Geometry check sheet. Reference: the model listing, model coordinates, mm. A direction names the side the tool comes from. Coordinates: 2 decimals unless noted, no trailing zeros. Write each loop counter-clockwise with the first axis right and the second up, starting at its lowest first coordinate (ties: lowest second). Pieces come first, ordered by that corner, then holes. Notation, with made-up numbers: (11, 37.25) - (18, 37.25) arc R27 cw to (18, 54.25) - close; hole circle Ø1 at (-24.5, 16). An arc over 180 degrees is marked (long way). Answer as a JSON object with one key per item and string values. Group by question number.
from build123d import *

# Parameters (mm, degrees)
SKETCH1_R           = 11.9
SKETCH1_W           = 2.4
SKETCH1_H           = 5
BOSS_EXTRUDE2_DEPTH = 2
SKETCH2_W           = 2.1
SKETCH2_H           = 2.4
BOSS_EXTRUDE3_DEPTH = 4.7
SKETCH4_W           = 2.1
SKETCH4_H           = 2.3
BOSS_EXTRUDE5_DEPTH = 1
SKETCH5_W           = 2.1
SKETCH5_H           = 2.3
BOSS_EXTRUDE6_DEPTH = 1
CHAMFER1_SIZE       = 1


with BuildPart() as part:
    # Sketch1 → Boss-Extrude2 (new body)
    with BuildSketch(Plane.XY):
        Circle(SKETCH1_R)
        with Locations((10, 0)):
            Rectangle(SKETCH1_W, SKETCH1_H, mode=Mode.SUBTRACT)
    extrude(amount=BOSS_EXTRUDE2_DEPTH)

    # Sketch2 → Boss-Extrude3 (add)
    with BuildSketch(Plane.XY.offset(2)):
        with Locations((-10, 0)):
            Rectangle(SKETCH2_W, SKETCH2_H)
    extrude(amount=BOSS_EXTRUDE3_DEPTH)

    # Sketch4 → Boss-Extrude5 (add)
    with BuildSketch(Plane(origin=(0, 1.2, 0), x_dir=(1, 0, 0), z_dir=(0, 1, 0))):
        with Locations((-10, -5.55)):
            Rectangle(SKETCH4_W, SKETCH4_H)
    extrude(amount=BOSS_EXTRUDE5_DEPTH)

    # Sketch5 → Boss-Extrude6 (add)
    with BuildSketch(Plane.XZ.offset(1.2)):
        with Locations((-10, 5.55)):
            Rectangle(SKETCH5_W, SKETCH5_H)
    extrude(amount=BOSS_EXTRUDE6_DEPTH)

    # Chamfer1
    chamfer1_edges = [part.edges().sort_by_distance(p)[0] for p in [
        (-8.95, 0, 6.7),
        (-11.05, 0, 6.7),
        (-10, 2.2, 6.7),
        (-10, -2.2, 6.7),
    ]]
    chamfer(chamfer1_edges, length=CHAMFER1_SIZE)


solid = part.part
(1) Section check C-C (x = 9.5). Record the cut outline in (y, z), and give its area (3 significant figures).
(2) Section check B-B (z = 1.25). Record the cut outline in (x, y).
(3) Section check D-D (x = 0). Record the cut outline in (y, z), and give its area (3 significant figures).
(4) Draft check along Z on faces 1 (the face through (-10, -2, 4.4)), 2 (the face through (-9.46, -0.03, 6.21)), 3 (the face through (8.8, 0, 1)). Enter one of: +Z half, -Z half, draft (parallel to the pull), parting line (faces both ways), or undercut.
(5) Material ranges on L1, parallel to Z at x = -3.5, y = 3; L2, parallel to Y at x = 0.25, z = 0.5; L3, parallel to X at y = -7.25, z = 1.75, recorded low to high. Write a range as [from, to].
(6) Set-up check for faces 4 (the face through (-10, -1.2, 3)), 5 (the face through (-11.05, 0, 4)), 6 (the face through (-8.95, 0, 4)): record each of +Z, -Z, +X, -X, +Y, -Y from which the full face is reachable in a straight line by a thin tool's end or side.
(7) Gauge pin test, flat ends, axial feed: pin 1 (1 mm diameter, centred on y = 1, z = 1, fed in from -X); pin 2 (2.5 mm diameter, centred on x = -9.5, z = 3, fed in from -Y); pin 3 (2 mm diameter, centred on x = 5, z = 2, fed in from -Y); pin 4 (2 mm diameter, centred on x = 8.5, z = 4.5, fed in from -Y). Record the tip position at first contact, or that the pin passes through.
(8) Section check A-A (y = 0). Record the cut outline in (x, z).
Conclusion:
{
 "1": {"outline": "(-7.17, 0) - (-2.5, 0) - (-2.5, 2) - (-7.17, 2) - close; (2.5, 0) - (7.17, 0) - (7.17, 2) - (2.5, 2) - close", "area": "18.7 mm^2"},
 "2": {"outline": "circle Ø23.8 at (0, 0); hole (8.8, -2.5) - (11.2, -2.5) - (11.2, 2.5) - (8.8, 2.5) - close"},
 "3": {"outline": "(-11.9, 0) - (11.9, 0) - (11.9, 2) - (-11.9, 2) - close", "area": "47.6 mm^2"},
 "4": {"face 1": "undercut", "face 2": "+Z half", "face 3": "draft"},
 "5": {"L1": "z = [0, 2]", "L2": "y = [-11.9, 11.9]", "L3": "x = [-9.44, 9.44]"},
 "6": {"face 4": "+X, -X, -Y", "face 5": "+Z, -X, +Y, -Y", "face 6": "+Z, +X, +Y, -Y"},
 "7": {"pin 1": "stops at x = -11.89", "pin 2": "stops at y = -8.07", "pin 3": "stops at y = -11.21", "pin 4": "passes through"},
 "8": {"outline": "(-11.9, 0) - (8.8, 0) - (8.8, 2) - (-8.95, 2) - (-8.95, 5.7) - (-9.95, 6.7) - (-10.05, 6.7) - (-11.05, 5.7) - (-11.05, 2) - (-11.9, 2) - close; (11.2, 0) - (11.9, 0) - (11.9, 2) - (11.2, 2) - close"}
}
